Work out the finished part from the listing and answer in its coordinate system (mm). Coordinates: 2 decimals unless noted, no trailing zeros. Order: outer loops, then holes, each group sorted by start corner. A loop starts at its lowest first (then second) coordinate and runs counter-clockwise, first axis right, second up. Notation, with made-up numbers: (51, 48.25) -> (106, 48.25) arc R20 cw to (106, 74.25) -> close; hole circle Ø6 at (41.25, 73). An arc over 180 degrees is marked (long way). Use one line per item in the form item = value.
from build123d import *

# Parameters (mm, degrees)
ESQUISSE1_R               = 1.5
ESQUISSE1_W               = 5.2
ESQUISSE1_H               = 3
T_LE_DE_BASE_PLI_E1_DEPTH = 3


# Sheet-metal steps are written as plain solids
with BuildPart() as part:
    # Esquisse1 → Tôle de base pliée1 (new body)
    with BuildSketch(Plane.XY):
        with BuildLine():
            Line((14.870524532, 15.712944318), (90.111215477, 14.728402402))
            ThreePointArc((90.111215477, 14.728402402), (93.812069805, 10.954190169), (90.062150056, 7.228723404))
            Line((90.062150056, 7.228723404), (15.334764804, 6.494002243))
            ThreePointArc((15.334764804, 6.494002243), (14.047901461, 6.312443531), (12.851298677, 5.805370946))
            ThreePointArc((12.851298677, 5.805370946), (3.813779457, 10.83890154), (12.606947349, 16.288064992))
            ThreePointArc((12.606947349, 16.288064992), (13.70468529, 15.866487084), (14.870524532, 15.712944318))
        make_face()
        with Locations((9.812150056, 10.978723404)):
            Circle(ESQUISSE1_R, mode=Mode.SUBTRACT)
        with Locations((90.062150056, 10.978723404)):
            Circle(ESQUISSE1_R, mode=Mode.SUBTRACT)
        with Locations((59.212150056, 10.978723404)):
            Rectangle(ESQUISSE1_W, ESQUISSE1_H, mode=Mode.SUBTRACT)
    extrude(amount=-T_LE_DE_BASE_PLI_E1_DEPTH)


solid = part.part
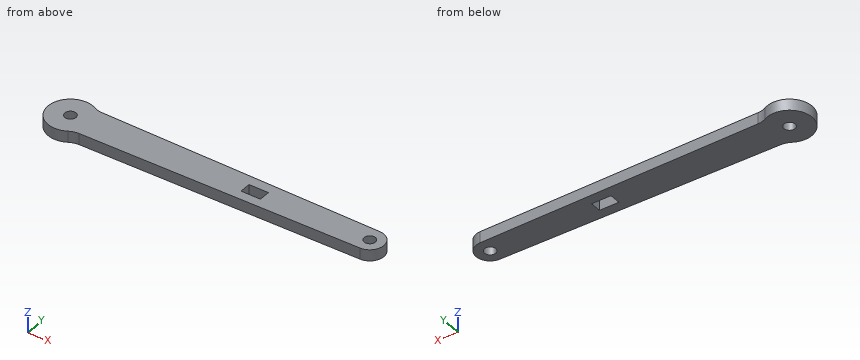
(1) Each of these flat-tipped pins is pushed along its axis until it touches: P1, Ø1, axis at y = 8, z = -2.5, coming from the -X side; P2, Ø1, axis at y = 13, z = -2, coming from the +X side. Where does it stop, or does it pass through?
Data:
P1 = 4.35
P2 = 93.49
(2) Section C-C on y = 8.5 is taken. Write down the section's boundary in (x, z), plus the area to 3 significant figures.
Data:
outline = (4.35, -3) -> (92.88, -3) -> (92.88, 0) -> (4.35, 0) -> close
area = 266 mm²
(3) Section B-B on x = 49 is taken. Write down the section's boundary in (y, z) (3 decimals), plus the area to 3 significant figures.
Data:
outline = (6.825, -3) -> (15.266, -3) -> (15.266, 0) -> (6.825, 0) -> close
area = 25.3 mm²
(4) Straight lines are drawn through the part: line 1 along X through (y, z) = (12.25, -1.05); line 2 along Y through (x, z) = (10, -0.6); line 3 along Y through (x, z) = (89.5, -0.5). For each, find the intervals that lie inside material, in ascending order.
Data:
line_1 = 3.95 to 9.02, 10.61 to 56.61, 61.81 to 89.27, 90.86 to 93.59
line_2 = 4.98 to 9.49, 12.47 to 16.98
line_3 = 7.22 to 9.59, 12.37 to 14.74
(5) Section A-A on z = -0.7 is taken. Write down the section's boundary in (x, y).
Data:
outline = (12.61, 16.29) arc R6 ccw (long way) to (12.85, 5.81) arc R5 cw to (15.33, 6.49) -> (90.06, 7.23) arc R3.75 ccw to (90.11, 14.73) -> (14.87, 15.71) arc R5 cw to start; hole circle Ø3 at (9.81, 10.98); hole (56.61, 9.48) -> (61.81, 9.48) -> (61.81, 12.48) -> (56.61, 12.48) -> close; hole circle Ø3 at (90.06, 10.98)
